Build history of the part. All positions in model axes, mm. Face numbers are marked on the shaded views. A direction names the side the tool comes from. Give positions to 0.01 mm unless a question says otherwise; leave off trailing zeros. Order: outer loops, then holes, each group sorted by start corner. A loop starts at its lowest first (then second) coordinate and runs counter-clockwise, first axis right, second up. Notation, with made-up numbers: M 40,66 L 77,66 A14 cw 77,88 Z; hole C -18,54 d3. An arc over 180 degrees is marked long. One line per item, written item: value.
Solid Edge part; units mm, degrees
sketch "Sketch1" plane through (0, 0, 0) normal (0, -1, 0) x (1, 0, 0)
  line L0 (-98.417, 1.7127) -> (11.583, 1.7127)
  line L1 (11.583, 1.7127) -> (11.583, 181.7127)
  line L2 (11.583, 181.7127) -> (-98.417, 181.7127)
  line L3 (-98.417, 181.7127) -> (-98.417, 1.7127)
  dimension "D1" = 98.417
  dimension "D2" = 98.417
extrude "Protrusion1" add sketch "Sketch1" against normal blind 10
sketch "Sketch2" plane through (-48.417, 0, 81.7127) normal (0, -1, 0) x (1, 0, 0)
  circle A0 centre (-36.5, 86.5) radius 5
  circle A1 centre (46.5, 86.5) radius 5
  circle A2 centre (-36.5, 3.5) radius 5
  circle A3 centre (46.5, 3.5) radius 5
  circle A4 centre (5, 45) radius 15
extrude "Cutout1" cut sketch "Sketch2" against normal through all
extrude "Cutout2" [suppressed]
sketch "Sketch3" plane through (-43.417, 10, 91.7127) normal (0, 1, 0) x (1, 0, 0)
  line L0 (-55, 90) -> (55, 90)
  line L1 (55, 90) -> (55, 80)
  line L2 (55, 80) -> (-55, 80)
  line L3 (-55, 80) -> (-55, 90)
  dimension "D1" = 55
extrude "Protrusion2" add sketch "Sketch3" along normal blind 100
sketch "Sketch4" plane through (-43.417, 60, 11.7127) normal (0, 0, 1) x (0, 1, 0)
  circle A0 centre (35, 30) radius 4
  circle A1 centre (-5, -30) radius 4
  circle A2 centre (35, -30) radius 4
  circle A3 centre (-5, 30) radius 4
  dimension "D1" = 35
extrude "Cutout3" cut sketch "Sketch4" against normal up to next
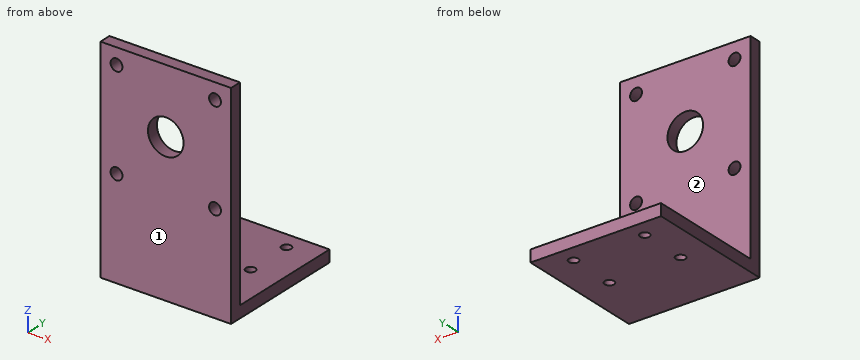
1) Saw through at C-C, the plane z = 23. Write the cut outline in (x, y), then the cut area to 3 significant figures.
Check values:
outline: M -98.42,0 L 11.58,0 L 11.58,10 L -98.42,10 Z
area: 1,100 mm^2
2) Saw through at D-D, the plane y = 22. Write the cut outline in (x, z).
Check values:
outline: M -98.42,1.71 L 11.58,1.71 L 11.58,11.71 L -98.42,11.71 Z
3) Pin check, flat tips, straight feed: pin 1 (1 mm diameter, centred on x = -20.5, z = 136, fed in from +Y); pin 2 (12 mm diameter, centred on x = -57.5, y = 84.5, fed in from +Z). Stop position of each tip, or through.
Check values:
pin 1: y = 10
pin 2: z = 11.71
4) Saw through at B-B, the plane x = -40.5. Write the cut outline in (y, z), then the cut area to 3 significant figures.
Check values:
outline: M 0,1.71 L 110,1.71 L 110,11.71 L 10,11.71 L 10,112 L 0,112 Z; M 0,141.43 L 10,141.43 L 10,181.71 L 0,181.71 Z
area: 2,510 mm^2
5) Drill centre lines: probe 1 along X at (y, z) = (95, 7); probe 2 along Z at (x, y) = (-1.5, 7); probe 3 along Z at (x, y) = (-8, 10.5). Where is each one in solid material? Low to high. Write a range as from..to.
Check values:
probe 1: -98.42..-77.42, -69.42..-17.42, -9.42..11.58
probe 2: 1.71..80.23, 90.2..163.23, 173.2..181.71
probe 3: 1.71..11.71
6) Tool access for the marked faces 1 and 2: list every direction of +Z, -Z, +X, -X, +Y, -Y with a clear straight run to the whole face (end or side of a thin tool).
Check values:
face 1: +Z, -Z, +X, -X, -Y
face 2: +Z, +X, -X, +Y
7) Saw through at A-A, the plane y = 55. Write the cut outline in (x, z), then the cut area to 3 significant figures.
Check values:
outline: M -98.42,1.71 L -77.42,1.71 L -77.42,11.71 L -98.42,11.71 Z; M -69.42,1.71 L -17.42,1.71 L -17.42,11.71 L -69.42,11.71 Z; M -9.42,1.71 L 11.58,1.71 L 11.58,11.71 L -9.42,11.71 Z
area: 940 mm^2
